from build123d import *

# Parameters (mm, degrees)
F1_DEPTH = 50
F1_TAPER = -57.2957795131
F2_T     = -2.5


with BuildPart() as f1:
    # F0 (on Top) → F1 (new body)
    with BuildSketch(Plane.XY):
        Polygon((86.2984904265, 0), (43.1492452133, 74.7366850176), (-43.1492452133, 74.7366850176), (-86.2984904265, 0), (-43.1492452133, -74.7366850176), (43.1492452133, -74.7366850176), align=None)
    extrude(amount=F1_DEPTH, taper=F1_TAPER)

    # F2
    f2_openings = [f1.faces().sort_by_distance(p)[0] for p in [
        (0, 0, 50),
    ]]
    offset(amount=F2_T, openings=f2_openings, kind=Kind.INTERSECTION)


solid = f1.part
Input: part model. Units: mm. Frame: model coordinates. A direction names the side the tool comes from. Give positions to 0.01 mm unless a question says otherwise; leave off trailing zeros. Write item = value, one per line. Start each with the question number.
1) First-contact query: pin 1 Ø12 at (y, z) = (0, 28.5) entering from +X; pin 2 Ø1.5 at (x, y) = (-2.5, -21.5) entering from +Z; pin 3 Ø10 at (x, z) = (-43, 11.5) entering from +Y. Flat tips, straight axial feed; report the tip coordinate or a pass-through.
2) Reachability of faces 1 (the flat face through (1, 1, 2.5)), 2 (the flat face through (-129.7, 79.8, 50)) from +Z, -Z, +X, -X, +Y, -Y: full face, straight path, thin tool, end or side. Return the list, or none.
3) Material intervals for line 1 along X through (y, z) = (45, 34); line 2 along X through (y, z) = (71.5, 28); line 3 along Z through (x, y) = (16, 45), sorted ascending. Write a range as [from, to].
Solved:
q1.pin_1 = 148.34
q1.pin_2 = 2.5
q1.pin_3 = 100.43
q2.face_1 = +Z
q2.face_2 = +Z, +X, -X, +Y, -Y
q3.line_1 = [-121.46, -116.12], [116.12, 121.46]
q3.line_2 = [-95.37, -90.03], [90.03, 95.37]
q3.line_3 = [0, 2.5]
